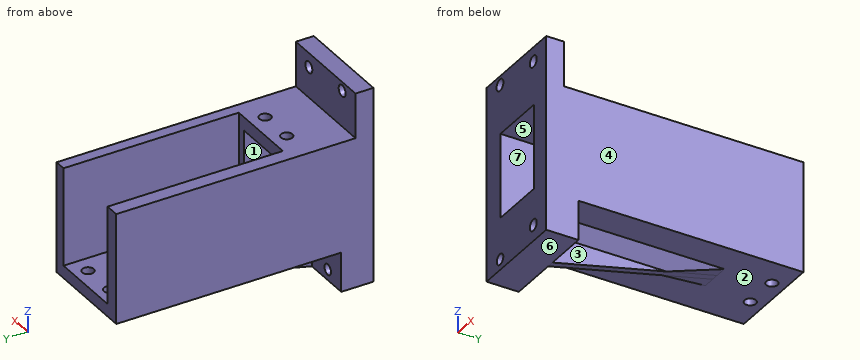
from build123d import *

# Parameters (mm, degrees)
SKETCH1_W               = 25
SKETCH1_H               = 17
BOSS_EXTRUDE1_DEPTH     = 12
MOVE_FACE1_BY           = 15
MOVE_FACE3_BY           = 8
SKETCH3_W               = 25
SKETCH3_H               = 12.751689795
BOSS_EXTRUDE2_DEPTH     = 6.9
SKETCH4_W               = 5
SKETCH4_H               = 16.698310205
BOSS_EXTRUDE3_DEPTH     = 6.9
MOVE_START              = -11.609792285
MOVE_FACE4_OUTLINE_W    = 6.9
MOVE_FACE4_OUTLINE_H    = 16.698310205
MOVE_FACE4_DEPTH        = 2.4
MOVE_FACE5_BY           = 20
SKETCH6_W               = 25
SKETCH6_H               = 10.9
BOSS_EXTRUDE5_DEPTH     = 2
MOVE_FACE6_BY           = 1.5
MOVE_FACE7_BY           = 2.6
SKETCH7_W               = 3.8
SKETCH7_H               = 30.95
BOSS_EXTRUDE6_DEPTH     = 41
SKETCH8_W               = 16.2
SKETCH8_H               = 3.5
BOSS_EXTRUDE7_DEPTH     = 41
SKETCH9_W               = 3
SKETCH9_H               = 30.95
BOSS_EXTRUDE8_DEPTH     = 41
SKETCH10_W              = 4.6
SKETCH10_H              = 3.5
BOSS_EXTRUDE9_DEPTH     = 41
MOVE_FACE8_BY           = 9
MOVE_FACE9_OUTLINE_W    = 6
MOVE_FACE9_OUTLINE_H    = 6.301689795
MOVE_FACE9_OUTLINE_H_2  = 3.5
MOVE_FACE9_DEPTH        = 27.6
MOVE_START_2            = 8.390207715
MOVE_FACE9_2_OUTLINE_W  = 6
MOVE_FACE9_2_OUTLINE_H  = 23.698310205
MOVE_FACE9_2_DEPTH      = 7.6
MOVE_FACE9_3_OUTLINE_W  = 6
MOVE_FACE9_3_OUTLINE_H  = 23.698310205
MOVE_FACE9_3_DEPTH      = 7.4
MOVE_FACE10_BY          = 10
SKETCH11_W              = 27.6
SKETCH11_H              = 3
BOSS_EXTRUDE10_DEPTH    = 11
SKETCH12_R              = 1.5
SKETCH12_R_2            = 1.6
CUT_EXTRUDE1_DEPTH      = 16
SKETCH13_R              = 1.6
CUT_EXTRUDE2_DEPTH      = 5
CUT_EXTRUDE3_START      = -9
SKETCH14_R              = 1.6
CUT_EXTRUDE3_DEPTH      = 9
SKETCH15_R              = 1.6
CUT_EXTRUDE4_DEPTH      = 5
MOVE_FACE14_BY          = 1
MOVE_FACE15_OUTLINE_W   = 16.9
MOVE_FACE15_OUTLINE_H   = 23.698310205
MOVE_FACE15_DEPTH       = 2
MOVE_FACE16_BY          = 8
MOVE_FACE17_BY          = 6
MOVE_FACE19_BY          = 6
MOVE_FACE20_BY          = 5
MOVE_FACE21_BY          = 0.2
MOVE_FACE22_BY          = 0.2
MOVE_START_3            = -12.454005935
MOVE_FACE23_OUTLINE_W   = 27.6
MOVE_FACE23_OUTLINE_H   = 62.9
MOVE_FACE23_DEPTH       = 0.05
MOVE_FACE24_BY          = 0.05
SKETCH17_R              = 1.6
CUT_EXTRUDE5_DEPTH      = 7.5
BOSS_EXTRUDE12_DEPTH    = 2
BOSS_EXTRUDE13_DEPTH    = 46
CUT_EXTRUDE6_DEPTH      = 70.24755409
CUT_EXTRUDE6_DEPTH_BACK = 70.24755409


# Read off the part's stored shape, not the designer's step: Move Face4, Move Face9, Move Face15, Move Face23
with BuildPart() as part:
    # Sketch1 → Boss-Extrude1 (new body)
    with BuildSketch(Plane(origin=(0, 0, 0), x_dir=(1, 0, 0), z_dir=(0, 1, 0))):
        with Locations((0.890207715, 2.454005935)):
            Rectangle(SKETCH1_W, SKETCH1_H)
    extrude(amount=BOSS_EXTRUDE1_DEPTH)

    # Move Face1: a face moved outward by 15.0
    extrude(part.faces().sort_by_distance((0.890207715, 6, 6.045994065))[0], amount=MOVE_FACE1_BY, dir=(0, 0, 1))

    # Move Face3: a face moved inward by 8.0
    extrude(part.faces().sort_by_distance((0.890207715, 12, 5.045994065))[0], amount=MOVE_FACE3_BY, dir=(0, -1, 0), mode=Mode.SUBTRACT)

    # Sketch3 → Boss-Extrude2 (add)
    with BuildSketch(Plane(origin=(0, 4, 0), x_dir=(1, 0, 0), z_dir=(0, 1, 0))):
        with Locations((0.890207715, -12.120149168)):
            Rectangle(SKETCH3_W, SKETCH3_H)
    extrude(amount=BOSS_EXTRUDE2_DEPTH)

    # Sketch4 → Boss-Extrude3 (add)
    with BuildSketch(Plane(origin=(0, 4, 0), x_dir=(1, 0, 0), z_dir=(0, 1, 0))):
        with Locations((10.890207715, 2.604850833)):
            Rectangle(SKETCH4_W, SKETCH4_H)
        with Locations((-6.709792285, 2.604850833)):
            Rectangle(SKETCH4_W, SKETCH4_H)
    extrude(amount=BOSS_EXTRUDE3_DEPTH)

    # Move Face4 outline → Move Face4 (add)
    with BuildSketch(Plane.YZ.offset(MOVE_START)):
        with Locations((7.45, -2.604850833)):
            Rectangle(MOVE_FACE4_OUTLINE_W, MOVE_FACE4_OUTLINE_H)
    extrude(amount=MOVE_FACE4_DEPTH)

    # Move Face5: a face moved inward by 20.0
    extrude(part.faces().sort_by_distance((2.090207715, 4, -2.604850832))[0], amount=MOVE_FACE5_BY, dir=(0, -1, 0), mode=Mode.SUBTRACT)

    # Sketch6 → Boss-Extrude5 (add)
    with BuildSketch(Plane(origin=(0, 0, -10.954005935), x_dir=(-1, 0, 0), z_dir=(0, 0, -1))):
        with Locations((-0.890207715, 5.45)):
            Rectangle(SKETCH6_W, SKETCH6_H)
    extrude(amount=-BOSS_EXTRUDE5_DEPTH)

    # Move Face6: a face moved outward by 1.5
    extrude(part.faces().sort_by_distance((0.890207715, 5.45, -10.954005935))[0], amount=MOVE_FACE6_BY, dir=(0, 0, -1))

    # Move Face7: a face moved outward by 2.6
    extrude(part.faces().sort_by_distance((13.390207715, 5.348749838, 3.512570938))[0], amount=MOVE_FACE7_BY, dir=(1, 0, 0))

    # Sketch7 → Boss-Extrude6 (add)
    with BuildSketch(Plane(origin=(0, 10.9, 0), x_dir=(1, 0, 0), z_dir=(0, 1, 0))):
        with Locations((-9.709792285, -3.020994065)):
            Rectangle(SKETCH7_W, SKETCH7_H)
    extrude(amount=BOSS_EXTRUDE6_DEPTH)

    # Sketch8 → Boss-Extrude7 (add)
    with BuildSketch(Plane(origin=(0, 10.9, 0), x_dir=(1, 0, 0), z_dir=(0, 1, 0))):
        with Locations((0.290207715, 10.704005935)):
            Rectangle(SKETCH8_W, SKETCH8_H)
    extrude(amount=BOSS_EXTRUDE7_DEPTH)

    # Sketch9 → Boss-Extrude8 (add)
    with BuildSketch(Plane(origin=(0, 10.9, 0), x_dir=(1, 0, 0), z_dir=(0, 1, 0))):
        with Locations((14.490207715, -3.020994065)):
            Rectangle(SKETCH9_W, SKETCH9_H)
    extrude(amount=BOSS_EXTRUDE8_DEPTH)

    # Sketch10 → Boss-Extrude9 (add)
    with BuildSketch(Plane(origin=(0, 10.9, 0), x_dir=(1, 0, 0), z_dir=(0, 1, 0))):
        with Locations((10.690207715, 10.704005935)):
            Rectangle(SKETCH10_W, SKETCH10_H)
    extrude(amount=BOSS_EXTRUDE9_DEPTH)

    # Move Face8: a face moved inward by 9.0
    extrude(part.faces().sort_by_distance((2.090207715, 5.45, 5.74430427))[0], amount=MOVE_FACE8_BY, dir=(0, 0, 1), mode=Mode.SUBTRACT)

    # Move Face9 outline → Move Face9 (add)
    with BuildSketch(Plane.YZ.offset(MOVE_START)):
        with Locations((-3, 17.895149168)):
            Rectangle(MOVE_FACE9_OUTLINE_W, MOVE_FACE9_OUTLINE_H)
        with Locations((-3, -10.704005935)):
            Rectangle(MOVE_FACE9_OUTLINE_W, MOVE_FACE9_OUTLINE_H_2)
    extrude(amount=MOVE_FACE9_DEPTH)

    # Move Face9 2 outline → Move Face9 2 (add)
    with BuildSketch(Plane.YZ.offset(MOVE_START_2)):
        with Locations((-3, 2.895149167)):
            Rectangle(MOVE_FACE9_2_OUTLINE_W, MOVE_FACE9_2_OUTLINE_H)
    extrude(amount=MOVE_FACE9_2_DEPTH)

    # Move Face9 3 outline → Move Face9 3 (add)
    with BuildSketch(Plane.YZ.offset(MOVE_START)):
        with Locations((-3, 2.895149167)):
            Rectangle(MOVE_FACE9_3_OUTLINE_W, MOVE_FACE9_3_OUTLINE_H)
    extrude(amount=MOVE_FACE9_3_DEPTH)

    # Move Face10: a face moved outward by 10.0
    extrude(part.faces().sort_by_distance((2.190207715, -1, 21.045994065))[0], amount=MOVE_FACE10_BY, dir=(0, 0, 1))

    # Sketch11 → Boss-Extrude10 (add)
    with BuildSketch(Plane(origin=(0, 0, -12.454005935), x_dir=(-1, 0, 0), z_dir=(0, 0, -1))):
        with Locations((-2.190207715, -4.5)):
            Rectangle(SKETCH11_W, SKETCH11_H)
    extrude(amount=BOSS_EXTRUDE10_DEPTH)

    # Sketch12 → Cut-Extrude1 (cut)
    with BuildSketch(Plane.XZ.offset(6)):
        with Locations(Location((-5.378312816, -20.454005935, 0), (0, 0, 270))):
            Circle(SKETCH12_R)
        with Locations(Location((-5.415791402, 28.545994065, 0), (0, 0, 270))):
            Circle(SKETCH12_R_2)
    extrude(amount=-CUT_EXTRUDE1_DEPTH, mode=Mode.SUBTRACT)

    # Sketch13 → Cut-Extrude2 (cut)
    with BuildSketch(Plane(origin=(0, -3, 0), x_dir=(1, 0, 0), z_dir=(0, 1, 0))):
        with Locations(Location((9.990207715, 18.954005935, 0), (0, 0, 180))):
            Circle(SKETCH13_R)
        with Locations(Location((9.990207715, -27.045994065, 0), (0, 0, 180))):
            Circle(SKETCH13_R)
    extrude(amount=-CUT_EXTRUDE2_DEPTH, mode=Mode.SUBTRACT)

    # Sketch14 → Cut-Extrude3 (cut)
    with BuildSketch(Plane.XZ.offset(3).offset(CUT_EXTRUDE3_START)):
        with Locations(Location((9.990207715, 27.045994065, 0), (0, 0, 90))):
            Circle(SKETCH14_R)
    extrude(amount=CUT_EXTRUDE3_DEPTH, mode=Mode.SUBTRACT)

    # Sketch15 → Cut-Extrude4 (cut)
    with BuildSketch(Plane.XY.offset(18.495994065)):
        with Locations((-2.209792285, 6.55)):
            Circle(SKETCH15_R)
        with Locations((7.790207715, 6.55)):
            Circle(SKETCH15_R)
    extrude(amount=-CUT_EXTRUDE4_DEPTH, mode=Mode.SUBTRACT)

    # Move Face14: a face moved inward by 1.0
    extrude(part.faces().sort_by_distance((-4.209792285, 2.45, 2.895149168))[0], amount=MOVE_FACE14_BY, dir=(-1, 0, 0), mode=Mode.SUBTRACT)

    # Move Face15 outline → Move Face15 (cut)
    with BuildSketch(Plane.YZ.offset(MOVE_START_2)):
        with Locations((2.45, 2.895149167)):
            Rectangle(MOVE_FACE15_OUTLINE_W, MOVE_FACE15_OUTLINE_H)
    extrude(amount=MOVE_FACE15_DEPTH, mode=Mode.SUBTRACT)

    # Move Face16: a face moved outward by 8.0
    extrude(part.faces().sort_by_distance((2.190207715, 51.9, -9.359005935))[0], amount=MOVE_FACE16_BY, dir=(0, 1, 0))

    # Move Face17: a face moved inward by 6.0
    extrude(part.faces().sort_by_distance((2.185483915, 4, 24.62368036))[0], amount=MOVE_FACE17_BY, dir=(0, -1, 0), mode=Mode.SUBTRACT)

    # Move Face19: a face moved outward by 6.0
    extrude(part.faces().sort_by_distance((13.230207715, -6, 3.795994065))[0], amount=MOVE_FACE19_BY, dir=(0, -1, 0))

    # Move Face20: a face moved inward by 5.0
    extrude(part.faces().sort_by_distance((2.185483915, -2, 24.62368036))[0], amount=MOVE_FACE20_BY, dir=(0, -1, 0), mode=Mode.SUBTRACT)

    # Move Face21: a face moved outward by 0.2
    extrude(part.faces().sort_by_distance((-7.809792285, 35.4, 4.770994065))[0], amount=MOVE_FACE21_BY, dir=(1, 0, 0))

    # Move Face22: a face moved outward by 0.2
    extrude(part.faces().sort_by_distance((12.990207715, 35.4, 4.770994065))[0], amount=MOVE_FACE22_BY, dir=(-1, 0, 0))

    # Move Face23 outline → Move Face23 (cut)
    with BuildSketch(Plane.XY.offset(MOVE_START_3)):
        with Locations((2.190207715, 28.45)):
            Rectangle(MOVE_FACE23_OUTLINE_W, MOVE_FACE23_OUTLINE_H)
    extrude(amount=MOVE_FACE23_DEPTH, mode=Mode.SUBTRACT)

    # Move Face24: a face moved outward by 0.05
    extrude(part.faces().sort_by_distance((2.590207715, 25.934788184, -8.954005935))[0], amount=MOVE_FACE24_BY, dir=(0, 0, 1))

    # Sketch17 → Cut-Extrude5 (cut)
    with BuildSketch(Plane.XY.offset(-8.904005935)):
        with Locations((-2.209792285, 56.05)):
            Circle(SKETCH17_R)
        with Locations((7.790207715, 56.05)):
            Circle(SKETCH17_R)
    extrude(amount=-CUT_EXTRUDE5_DEPTH, mode=Mode.SUBTRACT)

    # Sketch19 → Boss-Extrude12 (add)
    with BuildSketch(Plane(origin=(3.990207715, 0, 0), x_dir=(0, 0, -1), z_dir=(1, 0, 0))):
        Polygon((23.454005935, -3), (12.404005935, 43), (12.404005935, -3), align=None)
    extrude(amount=-BOSS_EXTRUDE12_DEPTH)

    # Sketch20 → Boss-Extrude13 (add)
    with BuildSketch(Plane(origin=(0, -3, 0), x_dir=(1, 0, 0), z_dir=(0, 1, 0))):
        Polygon((1.990207715, 15.804005935), (-1.409792285, 12.404005935), (1.990207715, 12.404005935), align=None)
        Polygon((3.990207715, 15.804005935), (7.390207715, 12.404005935), (3.990207715, 12.404005935), align=None)
    extrude(amount=BOSS_EXTRUDE13_DEPTH)

    # Sketch21 → Cut-Extrude6 (cut, two sides: drawn at the far end of the back side and taken through both)
    with BuildSketch(Plane(origin=(3.990207715, 0, 0), x_dir=(0, 0, -1), z_dir=(1, 0, 0)).offset(-CUT_EXTRUDE6_DEPTH_BACK)):
        Polygon((15.902869946, 28.434593255), (12.404005935, 43), (16.038201458, 43), align=None)
    extrude(amount=CUT_EXTRUDE6_DEPTH + CUT_EXTRUDE6_DEPTH_BACK, mode=Mode.SUBTRACT)


solid = part.part
Could you check a few things on this model? Use its own coordinates, in mm. Face numbers are marked on the shaded views. A direction names the side the tool comes from. Give positions to 0.01 mm unless a question says otherwise; leave off trailing zeros. Write each loop counter-clockwise with the first axis right and the second up, starting at its lowest first coordinate (ties: lowest second). Pieces come first, ordered by that corner, then holes. Notation, with made-up numbers: (-26.5, 74.5) -> (8.5, 74.5) arc R21 cw to (8.5, 89.5) -> close; hole circle Ø2 at (18, 20.5). An arc over 180 degrees is marked (long way). Answer as a JSON object with one key per item and string values.
Q1. We'd pull the mould along Z, two halves only. Please class the marked faces 4, 5, 6 and 7: released by +Z, released by -Z, zero draft, split by the parting line, or undercut.
Taken from the geometry:
{"face 4": "zero draft", "face 5": "undercut", "face 6": "released by -Z", "face 7": "undercut"}
Q2. Suppose I cut it at B-B on y = 56.05. Write out the boundary of the cut face in (x, z), then the cut area to 3 significant figures.
Taken from the geometry:
{"outline": "(-11.61, -12.4) -> (-3.81, -12.4) -> (-3.81, -8.9) -> (-7.61, -8.9) -> (-7.61, 18.5) -> (-11.61, 18.5) -> close; (-0.61, -12.4) -> (6.19, -12.4) -> (6.19, -8.9) -> (-0.61, -8.9) -> close; (9.39, -12.4) -> (15.99, -12.4) -> (15.99, 18.5) -> (12.79, 18.5) -> (12.79, -8.9) -> (9.39, -8.9) -> close", "area": "271 mm²"}
Q3. Suppose I cut it at A-A on z = -2. Write out the boundary of the cut face in (x, y), then the cut area to 3 significant figures.
Taken from the geometry:
{"outline": "(-11.61, -12) -> (-5.21, -12) -> (-5.21, 10.9) -> (-7.61, 10.9) -> (-7.61, 59.9) -> (-11.61, 59.9) -> close; (10.39, -12) -> (15.99, -12) -> (15.99, 59.9) -> (12.79, 59.9) -> (12.79, 10.9) -> (10.39, 10.9) -> close", "area": "628 mm²"}
Q4. Suppose I cut it at D-D on y = 6.55. Write out the boundary of the cut face in (x, z), then the cut area to 3 significant figures.
Taken from the geometry:
{"outline": "(-11.61, -12.4) -> (-1.41, -12.4) -> (1.99, -15.8) -> (1.99, -21.16) -> (3.99, -21.16) -> (3.99, -15.8) -> (7.39, -12.4) -> (15.99, -12.4) -> (15.99, 18.5) -> (9.39, 18.5) -> (9.39, 14.74) -> (10.39, 14.74) -> (10.39, -8.9) -> (-5.21, -8.9) -> (-5.21, 14.74) -> (-3.81, 14.74) -> (-3.81, 18.5) -> (-11.61, 18.5) -> close; (-0.61, 14.74) -> (6.19, 14.74) -> (6.19, 18.5) -> (-0.61, 18.5) -> close", "area": "489 mm²"}
Q5. Suppose I cut it at C-C on x = -9.5. Write out the boundary of the cut face in (y, z), then the cut area to 3 significant figures.
Taken from the geometry:
{"outline": "(-12, -23.45) -> (-3, -23.45) -> (-3, -12.4) -> (59.9, -12.4) -> (59.9, 18.5) -> (-7, 18.5) -> (-7, 31.05) -> (-12, 31.05) -> close", "area": "2,380 mm²"}
Q6. Which directions (+Z, -Z, +X, -X, +Y, -Y) give clear straight access to the entire face, cutting with the end or side of a thin tool? Please do the marked faces 1, 2 and 3.
Taken from the geometry:
{"face 1": "+Y, -Y", "face 2": "-Z, +Y", "face 3": "-Z, +X, +Y"}
Q7. Please list where these lines run through material, in increasing order: L1, parallel to X at y = 56, z = -11; L2, parallel to X at y = 33, z = 6; L3, parallel to Z at x = -2.5, y = 10.
Taken from the geometry:
{"L1": "x = -11.61 to -3.81, -0.61 to 6.19, 9.39 to 15.99", "L2": "x = -11.61 to -7.61, 12.79 to 15.99", "L3": "z = -12.4 to -8.9, 14.74 to 18.5"}
Q8. Will these pins go through, and if not, where does the flat tip stop? pin 1 Ø8.5 at (y, z) = (13, -21.5) entering from +X; pin 2 Ø10 at (x, z) = (-5, 24) entering from +Y; pin 3 Ø5.5 at (x, z) = (-2.5, -18.5) entering from +Y.
Taken from the geometry:
{"pin 1": "stops at x = 3.99", "pin 2": "stops at y = -7", "pin 3": "stops at y = -3"}
